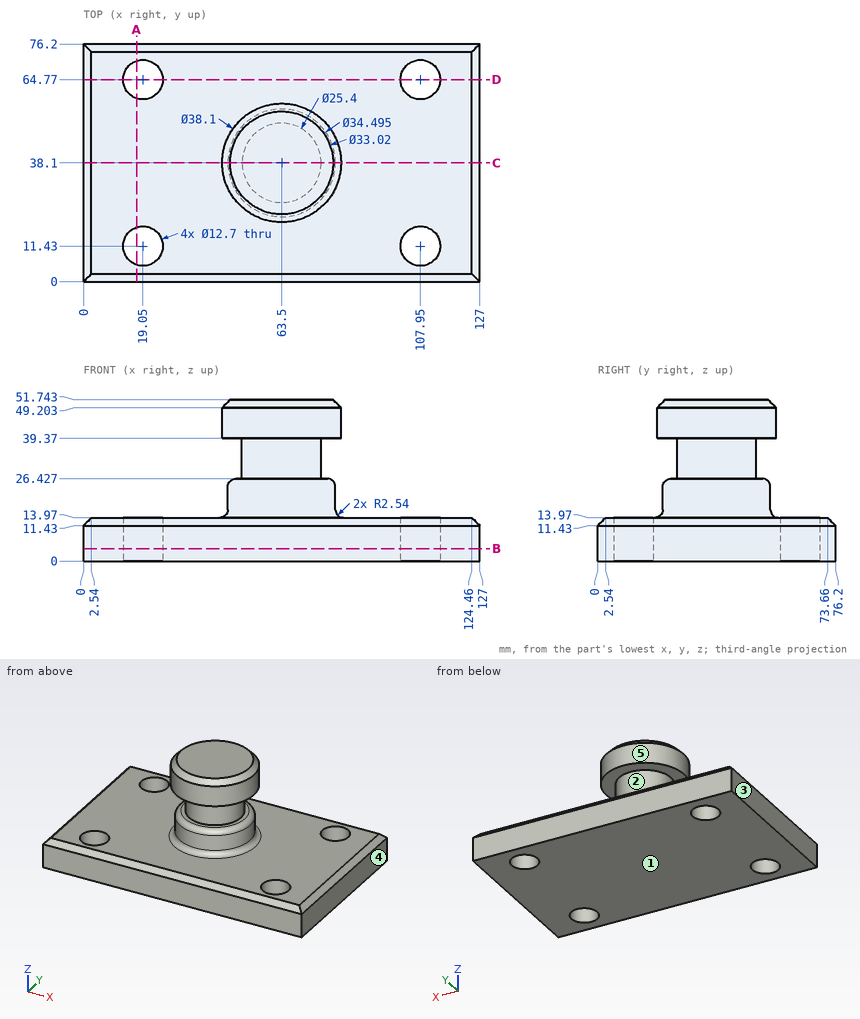
Job drawing, mm, ordinate dimensions from the low corner. One solid piece. A direction names the side the tool comes from. Coordinates: 2 decimals unless noted, no trailing zeros. Write each loop counter-clockwise with the first axis right and the second up, starting at its lowest first coordinate (ties: lowest second). Pieces come first, ordered by that corner, then holes. Notation, with made-up numbers: M 4.25,-37 L 62.25,-37 A18 cw 62.25,-15 Z; hole C 22.5,82 d4. An arc over 180 degrees is marked long. Answer as a JSON object with one key per item and string values. Group by question number.
1) Saw through at B-B (z = 4). Write the cut outline in (x, y), plus the area to 3 significant figures.
2) Pin check, flat tips, straight feed: pin 1 Ø10 at (x, y) = (105, 50.5) entering from +Z; pin 2 Ø8 at (y, z) = (31.5, 29) entering from -X; pin 3 Ø2 at (x, z) = (80.5, 21.5) entering from -Y. Stop position of each tip, or through.
3) Saw through at C-C (y = 38.1). Write the cut outline in (x, z), plus the area to 3 significant figures.
4) Tool access for the marked faces 4 and 5: list every direction of +Z, -Z, +X, -X, +Y, -Y with a clear straight run to the whole face (end or side of a thin tool).
5) Wall check: line 1 (Y direction, x = 19.05, z = 8); line 2 (X direction, y = 64, z = 7); line 3 (X direction, y = 63.5, z = 8.5). Give the ranges that are in metal, low to high. Write a range as from..to.
6) Saw through at D-D (y = 64.77). Write the cut outline in (x, z), plus the area to 3 significant figures.
7) Saw through at A-A (x = 17). Write the cut outline in (y, z).
8) Mould opens along Z. For the marked faces 1, 2 and 3 say: +Z half, -Z half, draft (parallel to the pull), parting line (faces both ways), or undercut.
Values follow:
{
 "1": {"outline": "M 0,0 L 127,0 L 127,76.2 L 0,76.2 Z; hole C 19.05,11.43 d12.7; hole C 19.05,64.77 d12.7; hole C 107.95,11.43 d12.7; hole C 107.95,64.77 d12.7", "area": "9,170 mm2"},
 "2": {"pin 1": "stops at z = 13.97", "pin 2": "stops at x = 47.47", "pin 3": "stops at y = 31.66"},
 "3": {"outline": "M 0,0 L 127,0 L 127,11.43 L 124.46,13.97 L 83.29,13.97 A2.54 cw 80.75,16.51 L 80.75,23.89 A2.54 ccw 78.21,26.43 L 76.2,26.43 L 76.2,39.37 L 82.55,39.37 L 82.55,49.2 L 80.01,51.74 L 46.99,51.74 L 44.45,49.2 L 44.45,39.37 L 50.8,39.37 L 50.8,26.43 L 48.79,26.43 A2.54 ccw 46.25,23.89 L 46.25,16.51 A2.54 cw 43.71,13.97 L 2.54,13.97 L 0,11.43 Z", "area": "2,990 mm2"},
 "4": {"face 4": "+Z, -Z, +X, +Y, -Y", "face 5": "+Z"},
 "5": {"line 1": "y = 0..5.08, 17.78..58.42, 71.12..76.2", "line 2": "x = 0..12.75, 25.35..101.65, 114.25..127", "line 3": "x = 0..12.83, 25.27..101.73, 114.17..127"},
 "6": {"outline": "M 0,0 L 12.7,0 L 12.7,13.97 L 2.54,13.97 L 0,11.43 Z; M 25.4,0 L 101.6,0 L 101.6,13.97 L 25.4,13.97 Z; M 114.3,0 L 127,0 L 127,11.43 L 124.46,13.97 L 114.3,13.97 Z", "area": "1,410 mm2"},
 "7": {"outline": "M 0,0 L 5.42,0 L 5.42,13.97 L 2.54,13.97 L 0,11.43 Z; M 17.44,0 L 58.76,0 L 58.76,13.97 L 17.44,13.97 Z; M 70.78,0 L 76.2,0 L 76.2,11.43 L 73.66,13.97 L 70.78,13.97 Z"},
 "8": {"face 1": "-Z half", "face 2": "undercut", "face 3": "draft"}
}
